from build123d import *

# Parameters (mm, degrees)
F0_R     = 50.7996215071
F1_DEPTH = 76.2
F1_TAPER = -15
F2_R     = 63.5
F3_DEPTH = 63.5
F3_TAPER = 15
F4_R     = 2.54
F5_R     = 12.7
F6_R     = 10.16


with BuildPart() as f1:
    # F0 (on Top) → F1 (new body)
    with BuildSketch(Plane.XY):
        Circle(F0_R)
    extrude(amount=F1_DEPTH, taper=F1_TAPER)

    # F2 (on face) → F3 (cut)
    with BuildSketch(Plane.XY.offset(76.2)):
        Circle(F2_R)
    extrude(amount=-F3_DEPTH, taper=F3_TAPER, mode=Mode.SUBTRACT)

    # F4
    f4_edges = [f1.edges().sort_by_distance(p)[0] for p in [
        (-71.21735, 0, 76.2),
        (-63.5, 0, 76.2),
    ]]
    fillet(f4_edges, radius=F4_R)

    # F5
    f5_edges = [f1.edges().sort_by_distance(p)[0] for p in [
        (-50.799622, 0, 0),
    ]]
    fillet(f5_edges, radius=F5_R)

    # F6
    f6_edges = [f1.edges().sort_by_distance(p)[0] for p in [
        (-46.485226, 0, 12.7),
    ]]
    fillet(f6_edges, radius=F6_R)


solid = f1.part
The model under review builds one solid part; all positions refer to its coordinate system, in mm. Coordinates: 2 decimals unless noted, no trailing zeros. Write each loop counter-clockwise with the first axis right and the second up, starting at its lowest first coordinate (ties: lowest second). Pieces come first, ordered by that corner, then holes. Notation, with made-up numbers: (-35.75, 87) - (-8.75, 87) arc R18 cw to (-8.75, 102) - close; hole circle Ø7 at (-6.75, 69). An arc over 180 degrees is marked (long way). Answer as a JSON object with one key per item and string values. Group by question number.
1. To check wall thickness, follow probe 1 along Z at (x, y) = (34.5, 4); probe 2 along X at (y, z) = (12, 13.5); probe 3 along X at (y, z) = (5, 38.5). State the ranges of each line that lie inside material, in increasing order.
2. Add section A-A (x = 0). Give the boundary of the cut face in (y, z), plus the area to 3 significant figures.
3. Clearance check with flat-ended pins moving along their axes: pin 1 Ø12 at (y, z) = (2.5, 39.5) entering from +X; pin 2 Ø5 at (x, y) = (-33.5, -51.5) entering from +Z; pin 3 Ø3 at (x, z) = (22.5, 34.5) entering from -Y. State where each tip first meets the part, or that it passes through.
4. Mouldability with a two-part tool opening along X and no side actions: class faces 1 (the face through (-12.61, -56.79, 27.52)), 2 (the face through (-1, 1, 0)), 3 (the face through (-1, 1, 12.7)), 4 (the face through (24.192, -46.512, 34.876)) as pulls with the +X half, pulls with the -X half, needs draft (parallel to the pull), parting line crosses it, or undercut.
5. Add section C-C (z = 60). Give the boundary of the cut face in (x, y).
6. Add section B-B (z = 68). Give the boundary of the cut face in (x, y), plus the area to 3 significant figures.
Findings:
{
 "1": {"probe 1": "0 to 12.7", "probe 2": "-53.08 to -40.92, 40.92 to 53.08", "probe 3": "-60.91 to -53.16, 53.16 to 60.91"},
 "2": {"outline": "(-70.36, 73) - (-53.32, 9.41) arc R12.7 ccw to (-41.05, 0) - (41.05, 0) arc R12.7 ccw to (53.32, 9.41) - (70.36, 73) arc R2.54 ccw to (67.91, 76.2) - (65.45, 76.2) arc R2.54 ccw to (63, 74.32) - (48.5, 20.23) arc R10.16 cw to (38.69, 12.7) - (-38.69, 12.7) arc R10.16 cw to (-48.5, 20.23) - (-63, 74.32) arc R2.54 ccw to (-65.45, 76.2) - (-67.91, 76.2) arc R2.54 ccw to start", "area": "2,290 mm²"},
 "3": {"pin 1": "x = 62.95", "pin 2": "z = 75.7", "pin 3": "y = -56.4"},
 "4": {"face 1": "parting line crosses it", "face 2": "needs draft", "face 3": "undercut", "face 4": "undercut"},
 "5": {"outline": "circle Ø133.75 at (0, 0); hole circle Ø118.32 at (0, 0)"},
 "6": {"outline": "circle Ø138.04 at (0, 0); hole circle Ø122.61 at (0, 0)", "area": "3,160 mm²"}
}
